```python
from build123d import *

# Parameters (mm, degrees)
SKETCH_R           = 57
PAD_DEPTH          = 3
SKETCH001_R        = 60.5
PAD001_DEPTH       = 3
CHAMFER_SIZE       = 0.5
CHAMFER001_SIZE    = 0.5
POCKET_DEPTH       = 2
POLARPATTERN_COUNT = 3
POLARPATTERN_ANGLE = 180
SKETCH003_W        = 2
SKETCH003_H        = 60.5
POCKET001_DEPTH    = 2
SKETCH004_W        = 2
SKETCH004_H        = 5
POCKET002_DEPTH    = 2
FILLET_R           = 3
FILLET001_R        = 1.5


with BuildPart() as part:
    # Sketch → Pad (new body)
    with BuildSketch(Plane.XY):
        Circle(SKETCH_R)
    extrude(amount=PAD_DEPTH)

    # Sketch001 (on Face2 of Pad) → Pad001 (join)
    with BuildSketch(Plane(origin=(0, 0, 0), x_dir=(1, 0, 0), z_dir=(0, 0, -1))):
        Circle(SKETCH001_R)
    extrude(amount=PAD001_DEPTH)

    # Chamfer
    chamfer_edges = [part.edges().sort_by_distance(p)[0] for p in [
        (-57, 0, 3),
    ]]
    chamfer(chamfer_edges, length=CHAMFER_SIZE)

    # Chamfer001
    chamfer001_edges = [part.edges().sort_by_distance(p)[0] for p in [
        (-60.5, 0, -3),
    ]]
    chamfer(chamfer001_edges, length=CHAMFER001_SIZE)

    # Sketch002 (on Face7 of Chamfer001) → Pocket (cut)
    with BuildSketch(Plane.XY.offset(3)):
        Polygon((-40, -1.5), (-40, 1.5), (-35, 1.5), (-35, 0.5), (0, 0.5), (0, -0.5), (-35, -0.5), (-35, -1.5), align=None)
    pocket = extrude(amount=-POCKET_DEPTH, mode=Mode.SUBTRACT)

    # PolarPattern: Pocket ×3 about axis
    polarpattern_axis = Axis((0, 0, 3), (0, 0, 1))
    for i in range(1, POLARPATTERN_COUNT):
        add(pocket.rotate(polarpattern_axis, i * POLARPATTERN_ANGLE / (POLARPATTERN_COUNT - 1)), mode=Mode.SUBTRACT)

    # Sketch003 (on Face7 of PolarPattern) → Pocket001 (cut)
    with BuildSketch(Plane.XY.offset(3)):
        with Locations((0, 30.25)):
            Rectangle(SKETCH003_W, SKETCH003_H)
    extrude(amount=-POCKET001_DEPTH, mode=Mode.SUBTRACT)

    # Sketch004 (on Face8 of Pocket001) → Pocket002 (cut)
    with BuildSketch(Plane.XY.offset(1)):
        with Locations((0, 58)):
            Rectangle(SKETCH004_W, SKETCH004_H)
    extrude(amount=-POCKET002_DEPTH, mode=Mode.SUBTRACT)

    # Fillet
    fillet_edges = [part.edges().sort_by_distance(p)[0] for p in [
        (1, 0.5, 2),
        (-1, 0.5, 2),
    ]]
    fillet(fillet_edges, radius=FILLET_R)

    # Fillet001
    fillet001_edges = [part.edges().sort_by_distance(p)[0] for p in [
        (0, 55.5, 1),
    ]]
    fillet(fillet001_edges, radius=FILLET001_R)


solid = part.part
```
CAD build for the part. Positions are in the model's coordinates, mm. A direction names the side the tool comes from. Round coordinates to 2 decimals unless told otherwise and drop trailing zeros. Write item = value, one per line. Start each with the question number.
Q1. Probe L1, parallel to Z at x = 50, y = -31; L2, parallel to X at y = -29, z = 1.4; L3, parallel to Y at x = 9, z = 2.05. List the from-to ranges inside material, lowest first. Write a range as from..to.
Q2. Which spindle directions (+Z, -Z, +X, -X, +Y, -Y) get a long thin tool onto all of the face, cutting with end or side? Do faces 1 (the flat face through (-1, 32, 2)), 2 (the cylindrical face through (-1.86, 1.4, 2.01)), 3 (the flat face through (-1, -12, 3)). Say none if no direction does.
Q3. Mould opens along X. For faces 4 (the flat face through (1, 32, 2)), 5 (the flat face through (-41, -41, 0)), 6 (the cylindrical face through (-13.12, 59.06, -1.23)) say: pulls with the +X half, pulls with the -X half, needs draft (parallel to the pull), parting line crosses it, or undercut.
Q4. Drop flat-ended pins along their axis: pin 1 (2 mm diameter, centred on y = -11, z = -0.5, fed in from +X); pin 2 (1.6 mm diameter, centred on x = -0.5, y = 58.5, fed in from +Z); pin 3 (1 mm diameter, centred on y = -21.5, z = 2.5, fed in from +X). Give the stop position or say it passes through.
Answers below:
q1.L1 = -3..0
q1.L2 = -49.07..-0.5, 0.5..49.07
q1.L3 = -56.28..-0.5, 0.5..56.28
q2.face_1 = +Z, +Y
q2.face_2 = +Z
q2.face_3 = +Z, +X, -X, +Y, -Y
q3.face_4 = undercut
q3.face_5 = needs draft
q3.face_6 = parting line crosses it
q4.pin_1 = 59.67
q4.pin_2 = 0
q4.pin_3 = 52.99
